from build123d import *

# Parameters (mm, degrees)
BOSS_EXTRUDE1_DEPTH = 7
SKETCH2_R           = 1.5
CUT_EXTRUDE3_DEPTH  = 7.5


with BuildPart() as part:
    # Sketch1 → Boss-Extrude1 (new body)
    with BuildSketch(Plane.XY):
        Polygon((0, 0), (60, -55), (60, -60), (40, -80), (53, -60), (53, -55), (-15, 0), align=None)
    extrude(amount=BOSS_EXTRUDE1_DEPTH)

    # Sketch2 → Cut-Extrude3 (cut, symmetric)
    with BuildSketch(Plane.XY.offset(7)):
        with Locations((-0.705610521, -5.582063241)):
            Circle(SKETCH2_R)
    extrude(amount=CUT_EXTRUDE3_DEPTH, both=True, mode=Mode.SUBTRACT)


solid = part.part
The listing builds one solid part. Answer for the finished solid, in the listing's coordinates (mm). A direction names the side the tool comes from. Coordinates: 2 decimals unless noted, no trailing zeros. Loops run counter-clockwise (first coordinate to the right, second up) from the corner with the lowest first, then second, coordinate; pieces in that order, holes last.
1) Determine the mould class of faces 1 (the face through (53, -58, 3)), 2 (the face through (46.41, -70.14, 3.45)), 3 (the face through (25, -31, 7)), 4 (the face through (-8, 0, 3)) for opening direction Y: pulls with the +Y half, pulls with the -Y half, needs draft (parallel to the pull), parting line crosses it, or undercut.
2) Find section A-A on x = 43. Write down the section's boundary in (y, z), then the cut area to 3 significant figures.
3) Find the intervals of material crossed by L1, parallel to Y at x = 52, z = 3.5; L2, parallel to X at y = -57, z = 5; L3, parallel to Y at x = 35, z = 6.25, in increasing order.
4) Find section C-C on y = -65. Write down the section's boundary in (x, z).
5) Find section B-B on z = 2.5. Write down the section's boundary in (x, y).
6) Find section D-D on x = 13.5. Write down the section's boundary in (y, z) (3 decimals), then the cut area to 3 significant figures.
7) Flat-ended cylindrical pins translate along their axes: pin 1 Ø2 at (y, z) = (-30, 1) entering from +X; pin 2 Ø1.5 at (x, z) = (24, 1) entering from +Y; pin 3 Ø2 at (y, z) = (-60.5, 1) entering from -X (3 decimals). Find the tip coordinate at first contact, or state that the pin passes through.
8) A tool of negligible diameter and unlimited length cuts with its end or side. For faces 5 (the face through (19.476, -27.885, 3.451)), 6 (the face through (25, -31, 0)), from which of +Z, -Z, +X, -X, +Y, -Y can it reach the whole face along a straight path? Write none if from no direction.
Values:
1. face 1: undercut
1. face 2: undercut
1. face 3: needs draft
1. face 4: pulls with the +Y half
2. outline: (-77, 0) - (-75.38, 0) - (-75.38, 7) - (-77, 7) - close; (-46.91, 0) - (-39.42, 0) - (-39.42, 7) - (-46.91, 7) - close
2. area: 63.8 mm2
3. L1: y = -68 to -61.54, -54.19 to -47.67
3. L2: x = 53 to 60
3. L3: y = -40.44 to -32.08
4. outline: (49.75, 0) - (55, 0) - (55, 7) - (49.75, 7) - close
5. outline: (-15, 0) - (53, -55) - (53, -60) - (40, -80) - (60, -60) - (60, -55) - (0, 0) - close; hole circle Ø3 at (-0.71, -5.58)
6. outline: (-23.051, 0) - (-12.375, 0) - (-12.375, 7) - (-23.051, 7) - close
6. area: 74.7 mm2
7. pin 1: stops at x = 33.82
7. pin 2: stops at y = -21.31
7. pin 3: stops at x = 52.025
8. face 5: +Z, -Z, -X
8. face 6: -Z, +X, -X, +Y, -Y
